The model under review builds one solid part; all positions refer to its coordinate system, in mm. A direction names the side the tool comes from. Coordinates: 2 decimals unless noted, no trailing zeros. Write each loop counter-clockwise with the first axis right and the second up, starting at its lowest first coordinate (ties: lowest second). Pieces come first, ordered by that corner, then holes.
1) Add section B-B, the plane z = -1.2. State the section outline as (x, y) points.
2) Add section D-D, the plane x = 1. State the section outline as (y, z) points.
3) Machinability: for faces 1 (the cylindrical face through (0.59, 4.08, 1.38)), 2 (the flat face through (0, 5, -1)), which of the approach directions +Z, -Z, +X, -X, +Y, -Y give a long, thin tool a straight path to every point of the face, cutting with its end or side? Answer none if there is none.
4) Add section C-C, the plane y = 0.75. State the section outline as (x, z) points.
5) Add section A-A, the plane x = 0. State the section outline as (y, z) points.
6) For line 1 (Y direction, x = 0.85, z = -1.05); line 2 (Z direction, x = 0.05, y = 2.25); line 3 (Z direction, x = -0.55, y = 5.25), list the stretches that pass through material, from the lowest coordinate up.
7) For P1, Ø1, axis at y = 2, z = 0.5, coming from the -X side; P2, Ø0.7, axis at x = -0.5, y = 5.5, coming from the -Z side, all flat-tipped, find the tip position at first contact; note any pin that passes through.
from build123d import *

# Parameters (mm, degrees)
SKETCH_1_R          = 1.5
EXTRUDE_1_DEPTH     = 10
CUT_EXTRUDE_1_DEPTH = 10
SKETCH1_R           = 1.5
BOSS_EXTRUDE1_DEPTH = 2


with BuildPart() as part:
    # Sketch 1 → Extrude 1 (new body)
    with BuildSketch(Plane(origin=(0, 0, 0), x_dir=(1, 0, 0), z_dir=(0, 1, 0))):
        Circle(SKETCH_1_R)
    extrude(amount=EXTRUDE_1_DEPTH)

    # Sketch 2 → Cut-Extrude 1 (cut)
    with BuildSketch(Plane(origin=(0, 10, 0), x_dir=(1, 0, 0), z_dir=(0, 1, 0))):
        with BuildLine():
            Line((-1.118033989, 1), (1.118033989, 1))
            ThreePointArc((1.118033989, 1), (0, 1.5), (-1.118033989, 1))
        make_face()
    extrude(amount=-CUT_EXTRUDE_1_DEPTH, mode=Mode.SUBTRACT)

    # Sketch1 → Boss-Extrude1 (add)
    with BuildSketch(Plane.XZ):
        Circle(SKETCH1_R)
    extrude(amount=BOSS_EXTRUDE1_DEPTH)


solid = part.part
Geometry results:
1. outline: (-0.9, -2) - (0.9, -2) - (0.9, 0) - (-0.9, 0) - close
2. outline: (-2, -1.12) - (0, -1.12) - (0, -1) - (10, -1) - (10, 1.12) - (-2, 1.12) - close
3. face 1: +Y, -Y
3. face 2: -Z, +X, -X, +Y
4. outline: (-1.12, -1) - (1.12, -1) arc R1.5 ccw (long way) to start
5. outline: (-2, -1.5) - (0, -1.5) - (0, -1) - (10, -1) - (10, 1.5) - (-2, 1.5) - close
6. line 1: y = -2 to 0
6. line 2: z = -1 to 1.5
6. line 3: z = -1 to 1.4
7. P1: stops at x = -1.5
7. P2: stops at z = -1
